from build123d import *

# Parameters (mm, degrees)
SKETCH1_W             = 6
SKETCH1_H             = 9.5
BOSS_EXTRUDE1_DEPTH   = 10
BOSS_EXTRUDE1_2_DEPTH = 10
SKETCH2_W             = 6
SKETCH2_H             = 6
CUT_EXTRUDE1_DEPTH    = 7
SKETCH3_W             = 28
SKETCH3_H             = 6
BOSS_EXTRUDE2_DEPTH   = 3
SKETCH4_R             = 1.5
CUT_EXTRUDE2_DEPTH    = 3
FILLET1_R             = 1
BOSS_EXTRUDE3_DEPTH   = 0.5
SKETCH6_R             = 1.1
CUT_EXTRUDE3_DEPTH    = 3


with BuildPart() as part:
    # Sketch1 → Boss-Extrude1 (new body)
    with BuildSketch(Plane.YZ):
        with Locations((233.5, -17.805567315)):
            Rectangle(SKETCH1_W, SKETCH1_H)
    extrude(amount=BOSS_EXTRUDE1_DEPTH)


with BuildPart() as body_2:
    # Sketch1 → Boss-Extrude1 2 (new body)
    with BuildSketch(Plane.YZ):
        with Locations((233.5, 12.694432685)):
            Rectangle(SKETCH1_W, SKETCH1_H)
    extrude(amount=BOSS_EXTRUDE1_2_DEPTH)


with BuildPart() as cut_extrude1_tool:
    # Sketch2 → Cut-Extrude1 (new body)
    with BuildSketch(Plane(origin=(10, 0, 0), x_dir=(0, 0, -1), z_dir=(1, 0, 0))):
        with Locations((-14.444432685, 233.5)):
            Rectangle(SKETCH2_W, SKETCH2_H)
        with Locations((19.555567315, 233.5)):
            Rectangle(SKETCH2_W, SKETCH2_H)
    extrude(amount=-CUT_EXTRUDE1_DEPTH)


with BuildPart() as part_1:
    add(part.part)

    # Cut-Extrude1: cut by cut_extrude1_tool
    add(cut_extrude1_tool.part, mode=Mode.SUBTRACT)



with BuildPart() as body_2_1:
    add(body_2.part)

    # Cut-Extrude1: cut by cut_extrude1_tool
    add(cut_extrude1_tool.part, mode=Mode.SUBTRACT)


with BuildPart() as part_2:
    add(part_1.part)

    add(body_2_1.part)  # Boss-Extrude2 merges body 2
    # Sketch3 → Boss-Extrude2 (add)
    with BuildSketch(Plane(origin=(10, 0, 0), x_dir=(0, 0, -1), z_dir=(1, 0, 0))):
        with Locations((2.555567315, 233.5)):
            Rectangle(SKETCH3_W, SKETCH3_H)
    extrude(amount=BOSS_EXTRUDE2_DEPTH)

    # Sketch4 → Cut-Extrude2 (cut)
    with BuildSketch(Plane.ZY.offset(-10)):
        with Locations((-8.055567315, 233.5)):
            Circle(SKETCH4_R)
        with Locations((2.944432685, 233.5)):
            Circle(SKETCH4_R)
    extrude(amount=-CUT_EXTRUDE2_DEPTH, mode=Mode.SUBTRACT)

    # Fillet1
    fillet1_edges = [part_2.edges().sort_by_distance(p)[0] for p in [
        (10, 233.5, -13.055567315),
        (3, 233.5, -16.555567315),
        (13, 233.5, 11.444432685),
        (13, 233.5, -16.555567315),
        (10, 233.5, 7.944432685),
        (3, 233.5, 11.444432685),
    ]]
    fillet(fillet1_edges, radius=FILLET1_R)

    # Sketch5 → Boss-Extrude3 (add, symmetric)
    with BuildSketch(Plane(origin=(0, 232.5, 0), x_dir=(-1, 0, 0), z_dir=(0, -1, 0))):
        Polygon((-12, 16.555567315), (-3, 20.055567315), (-3, 16.555567315), align=None)
        Polygon((-12, -11.444432685), (-3, -14.944432685), (-3, -11.444432685), align=None)
    extrude(amount=BOSS_EXTRUDE3_DEPTH, both=True)

    # Sketch6 → Cut-Extrude3 (cut)
    with BuildSketch(Plane(origin=(3, 0, 0), x_dir=(0, 0, -1), z_dir=(1, 0, 0))):
        with Locations((20.055567315, 234.5)):
            Circle(SKETCH6_R)
        with Locations((-14.944432685, 234.5)):
            Circle(SKETCH6_R)
    extrude(amount=-CUT_EXTRUDE3_DEPTH, mode=Mode.SUBTRACT)


solid = part_2.part
Read the model definition and answer for the solid it produces. Units are mm, in the model's axes. A direction names the side the tool comes from. Coordinates: 2 decimals unless noted, no trailing zeros. Loops run counter-clockwise (first coordinate to the right, second up) from the corner with the lowest first, then second, coordinate; pieces in that order, holes last. Notation, with made-up numbers: (5.5, 14.25) -> (51.5, 14.25) arc R30 cw to (51.5, 50.25) -> close; hole circle Ø7 at (26.5, -35.5). An arc over 180 degrees is marked (long way). Answer in a Markdown table with one row per item.
Item 1: A cutting plane is placed at A-A on x = 1.25. Determine the outline of the cut face in (y, z), plus the area to 3 significant figures.
Returned:
| item | result |
|---|---|
| outline | (230.5, -22.56) -> (236.5, -22.56) -> (236.5, -13.06) -> (230.5, -13.06) -> close; (230.5, 7.94) -> (236.5, 7.94) -> (236.5, 17.44) -> (230.5, 17.44) -> close; hole circle Ø2.2 at (234.5, -20.06); hole circle Ø2.2 at (234.5, 14.94) |
| area | 106 mm^2 |
Item 2: Each of these flat-tipped pins is pushed along its axis until it touches: P1, Ø1.8, axis at x = 7.5, y = 234.5, coming from the +Z side; P2, Ø0.8, axis at x = 9, y = 231.5, coming from the -Z side; P3, Ø1.3, axis at y = 234.5, z = 14.94, coming from the +X side; P4, Ø1.8, axis at x = 7, z = -19, coming from the +Y side. Where does it stop, or does it pass through?
Returned:
| item | result |
|---|---|
| P1 | stops at z = 11.44 |
| P2 | stops at z = -16.56 |
| P3 | passes through |
| P4 | stops at y = 233 |
Item 3: For faces 1 (the flat face through (8, 231, -16.556)), 2 (the flat face through (3, 233, 16)), 3 (the cylindrical face through (9.7, 233.54, -12.77)), determine the directions among +Z, -Z, +X, -X, +Y, -Y from which every point of the face is accessible in a straight line to the end or side of a thin tool.
Returned:
| item | result |
|---|---|
| face 1 | -Z, +X, -Y |
| face 2 | +Z, +X |
| face 3 | -X, +Y, -Y |
Item 4: A cutting plane is placed at D-D on x = 7.25. Determine the outline of the cut face in (y, z), plus the area to 3 significant figures.
Returned:
| item | result |
|---|---|
| outline | (230.5, -16.56) -> (232, -16.56) -> (232, -18.4) -> (233, -18.4) -> (233, -16.56) -> (236.5, -16.56) -> (236.5, -13.06) -> (230.5, -13.06) -> close; (230.5, 7.94) -> (236.5, 7.94) -> (236.5, 11.44) -> (233, 11.44) -> (233, 13.29) -> (232, 13.29) -> (232, 11.44) -> (230.5, 11.44) -> close |
| area | 45.7 mm^2 |
Item 5: A cutting plane is placed at C-C on y = 234.5. Give the number of separate pieces and of enclosed holes in the cut face, plus the area to 3 significant figures.
Returned:
| item | result |
|---|---|
| separate pieces | 5 |
| enclosed holes | 0 |
| area | 164 mm^2 |
Item 6: For a pull along Y with two mould halves and no side action, classify faces 4 (the cylindrical face through (3.3, 234.77, 11.73)), 5 (the cylindrical face through (1.521, 233.524, 14.437)), 6 (the flat face through (5, 232, -18)), 7 (the flat face through (6, 233, 12)) as released by +Y, released by -Y, zero draft, split by the parting line, or undercut.
Returned:
| item | result |
|---|---|
| face 4 | zero draft |
| face 5 | undercut |
| face 6 | released by -Y |
| face 7 | released by +Y |
Item 7: Straight lines are drawn through the part: line 1 along Z through (x, y) = (2.05, 234.5); line 2 along Z through (x, y) = (12.1, 233.5); line 3 along Z through (x, y) = (6.25, 235.25). For each, find the intervals that lie inside material, in ascending order. Write a range as [from, to].
Returned:
| item | result |
|---|---|
| line 1 | z = [-22.56, -21.16], [-18.96, -13.06], [7.94, 13.84], [16.04, 17.44] |
| line 2 | z = [-16.55, -9.56], [-6.56, 1.44], [4.44, 11.44] |
| line 3 | z = [-16.56, -13.06], [7.94, 11.44] |
Item 8: A cutting plane is placed at B-B on y = 231. Determine the outline of the cut face in (x, z), plus the area to 3 significant figures.
Returned:
| item | result |
|---|---|
| outline | (0, -22.56) -> (3, -22.56) -> (3, -17.56) arc R1 cw to (4, -16.56) -> (12, -16.56) arc R1 ccw to (13, -15.56) -> (13, 10.44) arc R1 ccw to (12, 11.44) -> (4, 11.44) arc R1 cw to (3, 12.44) -> (3, 17.44) -> (0, 17.44) -> (0, 7.94) -> (9, 7.94) arc R1 cw to (10, 6.94) -> (10, -12.06) arc R1 cw to (9, -13.06) -> (0, -13.06) -> close |
| area | 190 mm^2 |
